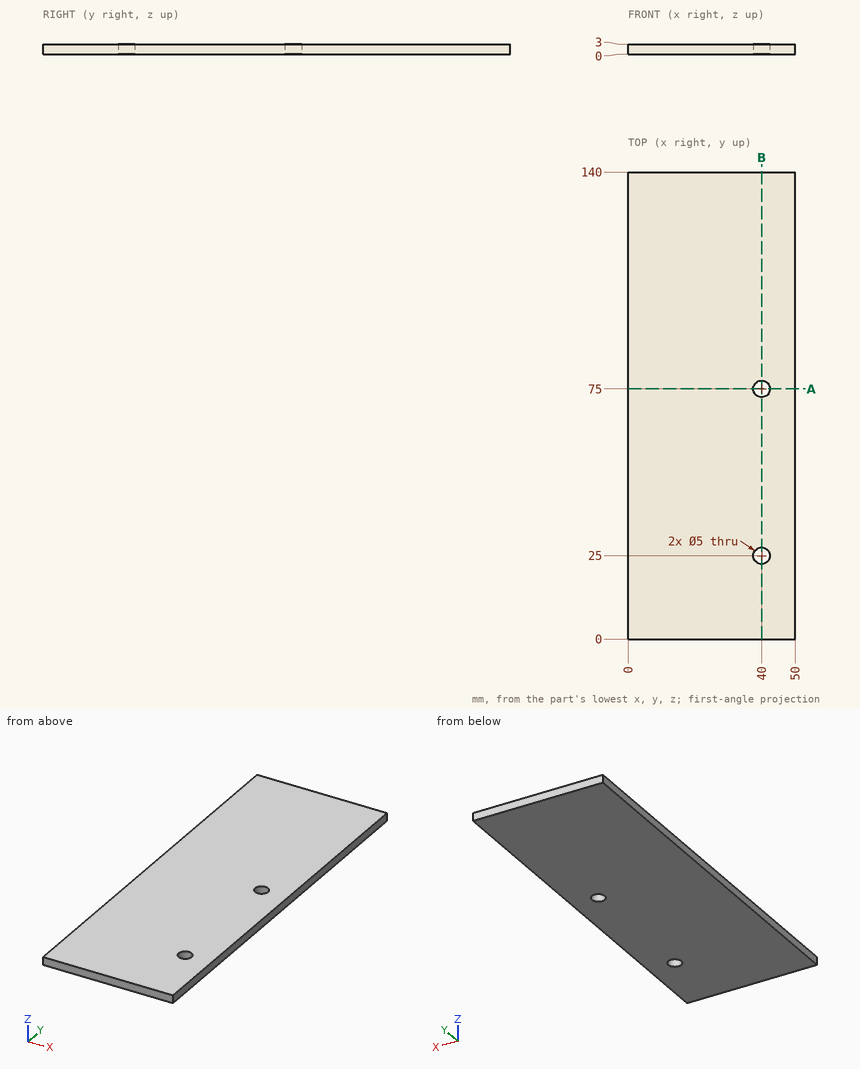
Design review of the part shown in the three views and the two pictorial views. Dimensions are in mm from the part's minimum x, y and z. Round coordinates to 2 decimals unless told otherwise and drop trailing zeros. Order: outer loops, then holes, each group sorted by start corner. A loop starts at its lowest first (then second) coordinate and runs counter-clockwise, first axis right, second up. Notation, with made-up numbers: (40, 78.5) -> (89, 78.5) arc R25 cw to (89, 97.5) -> close; hole circle Ø4 at (78.5, 29). An arc over 180 degrees is marked (long way). Write item = value, one per line. Start each with the question number.
1) Take a section at B-B on x = 40. State the section outline as (y, z) points, plus the area to 3 significant figures.
2) To check wall thickness, follow line 1 (Y direction, x = 40, z = 0.75); line 2 (Y direction, x = 38.5, z = 1.5); line 3 (X direction, y = 77, z = 0.6). State the ranges of each line that lie inside material, in increasing order. Write a range as from..to.
3) Take a section at A-A on y = 75. State the section outline as (x, z) points.
Verdict:
q1.outline = (0, 0) -> (22.5, 0) -> (22.5, 3) -> (0, 3) -> close; (27.5, 0) -> (72.5, 0) -> (72.5, 3) -> (27.5, 3) -> close; (77.5, 0) -> (140, 0) -> (140, 3) -> (77.5, 3) -> close
q1.area = 390 mm2
q2.line_1 = 0..22.5, 27.5..72.5, 77.5..140
q2.line_2 = 0..23, 27..73, 77..140
q2.line_3 = 0..38.5, 41.5..50
q3.outline = (0, 0) -> (37.5, 0) -> (37.5, 3) -> (0, 3) -> close; (42.5, 0) -> (50, 0) -> (50, 3) -> (42.5, 3) -> close
